Part model, mm, in its own coordinate system. Face numbers are marked on the shaded views. A direction names the side the tool comes from. Round coordinates to 2 decimals unless told otherwise and drop trailing zeros. Loops run counter-clockwise (first coordinate to the right, second up) from the corner with the lowest first, then second, coordinate; pieces in that order, holes last.
from build123d import *

# Parameters (mm, degrees)
F0_W     = 140.959114
F0_H     = 71.438462
F1_DEPTH = 304.8
F2_W     = 119.863194
F2_H     = 233.014038
F3_DEPTH = 152.4
F4_W     = 35.95896
F4_H     = 35.000048
F5_DEPTH = 254
F6_R     = 11.870693
F7_DEPTH = 304.8


with BuildPart() as f1:
    # F0 (on Front) → F1 (new body)
    with BuildSketch(Plane.XZ):
        Rectangle(F0_W, F0_H)
    extrude(amount=F1_DEPTH)

    # F2 (on Top) → F3 (cut)
    with BuildSketch(Plane.XY):
        with Locations((-0.958899, -124.89744)):
            Rectangle(F2_W, F2_H)
    extrude(amount=-F3_DEPTH, mode=Mode.SUBTRACT)

    # F4 (on Top) → F5 (cut)
    with BuildSketch(Plane.XY):
        with Locations((45.068562, -29.9658)):
            Rectangle(F4_W, F4_H)
    extrude(amount=-F5_DEPTH, mode=Mode.SUBTRACT)

    # F6 (on Front) → F7 (cut)
    with BuildSketch(Plane.XZ):
        with Locations((-40.513758, 16.780848)):
            Circle(F6_R)
    extrude(amount=-F7_DEPTH, mode=Mode.SUBTRACT)


solid = f1.part
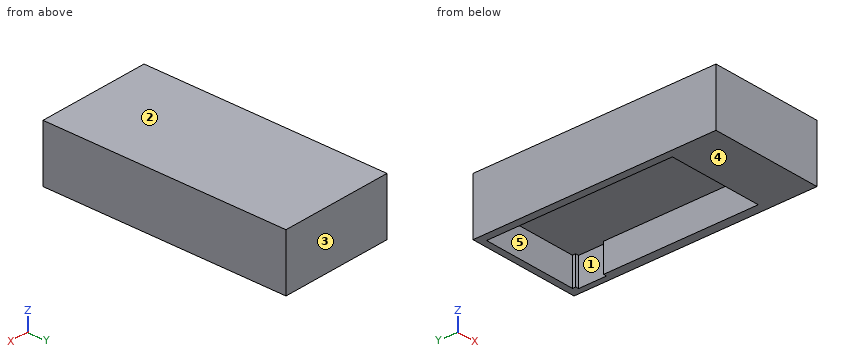
1) Slice it at C-C, the plane z = -6. Give the cut face in (x, y).
Values:
outline: (-70.48, -304.8) - (70.48, -304.8) - (70.48, 0) - (-70.48, 0) - close; hole (-60.89, -241.4) - (58.97, -241.4) - (58.97, -47.47) - (63.05, -47.47) - (63.05, -12.47) - (58.97, -12.47) - (58.97, -8.39) - (-60.89, -8.39) - close
2) Drop a flat-ended pin along its axis: pin 1 Ø4 at (x, y) = (-36, -62) entering from -Z. Give the stop position or say it passes through.
Values:
pin 1: stops at z = 0
3) Slice it at B-B, the plane y = -232.5. Give the cut face in (x, z), then the cut area to 3 significant figures.
Values:
outline: (-70.48, -35.72) - (-60.89, -35.72) - (-60.89, 0) - (58.97, 0) - (58.97, -35.72) - (70.48, -35.72) - (70.48, 35.72) - (-70.48, 35.72) - close
area: 5,790 mm2
4) Tool access for the marked faces 4 and 5: list every direction of +Z, -Z, +X, -X, +Y, -Y with a clear straight run to the whole face (end or side of a thin tool).
Values:
face 4: -Z, +X, -X, +Y, -Y
face 5: -Z
5) Wall check: line 1 along Y through (x, z) = (-25.5, -9.5); line 2 along X through (y, z) = (-75, -1); line 3 along X through (y, z) = (-20, -13). Give the ranges that are in metal, low to high.
Values:
line 1: y = -304.8 to -241.4, -8.39 to 0
line 2: x = -70.48 to -60.89, 58.97 to 70.48
line 3: x = -70.48 to -60.89, 63.05 to 70.48
6) Slice it at A-A, the plane x = -42.5. Give the cut face in (y, z), then the cut area to 3 significant figures.
Values:
outline: (-304.8, -35.72) - (-241.4, -35.72) - (-241.4, 0) - (-8.39, 0) - (-8.39, -35.72) - (0, -35.72) - (0, 35.72) - (-304.8, 35.72) - close
area: 13,500 mm2
7) Mould opens along Y. For the marked faces 1, 2 and 3 say: released by +Y, released by -Y, zero draft, split by the parting line, or undercut.
Values:
face 1: undercut
face 2: zero draft
face 3: released by +Y
